Here's how the part is built. I have some questions about the finished solid (model axes, mm). A direction names the side the tool comes from. Round coordinates to 2 decimals unless told otherwise and drop trailing zeros. Order: outer loops, then holes, each group sorted by start corner. A loop starts at its lowest first (then second) coordinate and runs counter-clockwise, first axis right, second up. Notation, with made-up numbers: (40.25, 76.25) - (62.25, 76.25) arc R20 cw to (62.25, 105.25) - close; hole circle Ø8 at (75, 5.25). An arc over 180 degrees is marked (long way). One line per item, written item: value.
from build123d import *

# Parameters (mm, degrees)
F0_W          = 30.0000000298
F0_H          = 57.0000000298
F0_W_2        = 20
F0_H_2        = 47
F1_DEPTH      = 70
F1_DEPTH_BACK = 70
F2_R          = 5
F3_W          = 10.0000004768
F3_H          = 37.0000004768
F4_DEPTH      = 120
F5_R          = 5
F6_R          = 2.074
F7_DEPTH      = 20


with BuildPart() as f1:
    # F0 (on Top) → F1 (new body, two sides)
    with BuildSketch(Plane.XY) as f1_sk:
        Rectangle(F0_W, F0_H)
        Rectangle(F0_W_2, F0_H_2, mode=Mode.SUBTRACT)
    extrude(amount=F1_DEPTH)
    extrude(f1_sk.sketch, amount=-F1_DEPTH_BACK)

    # F2
    f2_edges = [f1.edges().sort_by_distance(p)[0] for p in [
        (-10, 23.5, 0),
        (10, 23.5, 0),
        (-10, -23.5, 0),
        (10, -23.5, 0),
        (-15, 28.5, 0),
        (15, 28.5, 0),
        (15, -28.5, 0),
        (-15, -28.5, 0),
    ]]
    fillet(f2_edges, radius=F2_R)

    # F3 (on face) → F4 (join)
    with BuildSketch(Plane(origin=(0, 0, -70), x_dir=(1, 0, 0), z_dir=(0, 0, -1))):
        with BuildLine():
            Line((-10, 18.5), (-10, -18.5))
            ThreePointArc((-10, -18.5), (-8.5355339059, -22.0355339059), (-5, -23.5))
            Line((-5, -23.5), (5, -23.5))
            ThreePointArc((5, -23.5), (8.5355339059, -22.0355339059), (10, -18.5))
            Line((10, -18.5), (10, 18.5))
            ThreePointArc((10, 18.5), (8.5355339059, 22.0355339059), (5, 23.5))
            Line((5, 23.5), (-5, 23.5))
            ThreePointArc((-5, 23.5), (-8.5355339059, 22.0355339059), (-10, 18.5))
        make_face()
        Rectangle(F3_W, F3_H, mode=Mode.SUBTRACT)
    extrude(amount=-F4_DEPTH)

    # F5
    f5_edges = [f1.edges().sort_by_distance(p)[0] for p in [
        (-5, -18.5, -10),
        (5, -18.5, -10),
        (5, 18.5, -10),
        (-5, 18.5, -10),
    ]]
    fillet(f5_edges, radius=F5_R)

    # F6 (on face) → F7 (cut)
    with BuildSketch(Plane(origin=(0, 0, -70), x_dir=(1, 0, 0), z_dir=(0, 0, -1))):
        with Locations((-10.0000000149, 23.5000000149)):
            Circle(F6_R)
        with Locations((10.0000000149, 23.5000000149)):
            Circle(F6_R)
        with Locations((-10.0000000149, -23.5000000149)):
            Circle(F6_R)
        with Locations((10.0000000149, -23.5000000149)):
            Circle(F6_R)
    extrude(amount=-F7_DEPTH, mode=Mode.SUBTRACT)


solid = f1.part
Q1. We'd pull the mould along Y, two halves only. Please class faces 6 (the cylindrical face through (8.57, -22, 59.86)), 7 (the cylindrical face through (-13.57, 27, -0.98)), 8 (the flat face through (-10.2, 0.4, 70)): released by +Y, released by -Y, zero draft, split by the parting line, or undercut.
Results list:
face 6: undercut
face 7: released by +Y
face 8: zero draft
Q2. If we section it at C-C, the plane y = -20: Please give me the cut outline in (x, z).
Results list:
outline: (-15, -70) - (15, -70) - (15, 70) - (9.77, 70) - (9.77, 50) - (-9.77, 50) - (-9.77, 70) - (-15, 70) - close
Q3. If we section it at B-B, the plane z = -10: Please give me the cut outline in (x, y).
Results list:
outline: (-15, -23.5) arc R5 ccw to (-10, -28.5) - (10, -28.5) arc R5 ccw to (15, -23.5) - (15, 23.5) arc R5 ccw to (10, 28.5) - (-10, 28.5) arc R5 ccw to (-15, 23.5) - close; hole (-5, -13.5) arc R5 ccw to (5, -13.5) - (5, 13.5) arc R5 ccw to (-5, 13.5) - close
Q4. If we section it at A-A, the plane y = 4: Please give me the cut outline in (x, z), then the cut area to 3 significant figures.
Results list:
outline: (-15, -70) - (-5, -70) - (-5, 50) - (-10, 50) - (-10, 70) - (-15, 70) - close; (5, -70) - (15, -70) - (15, 70) - (10, 70) - (10, 50) - (5, 50) - close
area: 2,600 mm²
Q5. Which directions (+Z, -Z, +X, -X, +Y, -Y) give clear straight access to the entire face, cutting with the end or side of a thin tool? Please do faces 1 (the cylindrical face through (8.5, 22.07, 59.86)), 2 (the flat face through (6, 0, -70)), 3 (the flat face through (10, 23, -50)), 4 (the flat face through (0, 28.5, 1)), 5 (the flat face through (-5, 0, -11)).
Results list:
face 1: +Z
face 2: -Z, +X, -X, +Y, -Y
face 3: -Z
face 4: +Z, -Z, +X, -X, +Y
face 5: +Z, -Z
Q6. Will these pins go through, and if not, where does the flat tip stop? pin 1 (10 mm diameter, centred on x = -2, y = -1.5, fed in from +Z); pin 2 (2.5 mm diameter, centred on x = 10, y = 23.5, fed in from -Z).
Results list:
pin 1: z = 50
pin 2: z = -50
Q7. If we section it at D-D, the plane z = 59: Please give me the cut outline in (x, y).
Results list:
outline: (-15, -23.5) arc R5 ccw to (-10, -28.5) - (10, -28.5) arc R5 ccw to (15, -23.5) - (15, 23.5) arc R5 ccw to (10, 28.5) - (-10, 28.5) arc R5 ccw to (-15, 23.5) - close; hole (-10, -18.5) arc R5 ccw to (-5, -23.5) - (5, -23.5) arc R5 ccw to (10, -18.5) - (10, 18.5) arc R5 ccw to (5, 23.5) - (-5, 23.5) arc R5 ccw to (-10, 18.5) - close
Q8. If I drill on line 1 along Y through (x, z) = (-10, -61); line 2 along X through (y, z) = (-23.5, -64.5); line 3 along X through (y, z) = (23, -55), over which ranges is the centre line in solid material (lowest first)?
Results list:
line 1: -28.5 to -25.57, -21.43 to 21.43, 25.57 to 28.5
line 2: -15 to -12.07, -7.93 to 7.93, 12.07 to 15
line 3: -15 to -12.01, -7.99 to 7.99, 12.01 to 15
